```python
from build123d import *

# Parameters (mm, degrees)
SKETCH1_R           = 2.4892
BOSS_EXTRUDE1_DEPTH = 33.3375
CUT_EXTRUDE2_DEPTH  = 7.9375


with BuildPart() as part:
    # Sketch1 → Boss-Extrude1 (new, symmetric)
    with BuildSketch(Plane.XY):
        with BuildLine():
            ThreePointArc((-2.634980936, 6.35), (-3.437499983, 5.953924622), (-4.181770846, 5.456960429))
            Line((-4.181770846, 5.456960429), (-6.816751782, 0.893039571))
            ThreePointArc((-6.816751782, 0.893039571), (-6.874999966, 0), (-6.816751782, -0.893039571))
            Line((-6.816751782, -0.893039571), (-4.181770846, -5.456960429))
            ThreePointArc((-4.181770846, -5.456960429), (-3.437499983, -5.953924622), (-2.634980936, -6.35))
            Line((-2.634980936, -6.35), (2.634980936, -6.35))
            ThreePointArc((2.634980936, -6.35), (3.437499983, -5.953924622), (4.181770846, -5.456960429))
            Line((4.181770846, -5.456960429), (6.816751782, -0.893039571))
            ThreePointArc((6.816751782, -0.893039571), (6.860422465, -0.447468582), (6.874999966, 0))
            ThreePointArc((6.874999966, 0), (6.860422465, 0.447468582), (6.816751782, 0.893039571))
            Line((6.816751782, 0.893039571), (4.181770846, 5.456960429))
            ThreePointArc((4.181770846, 5.456960429), (3.437499983, 5.953924622), (2.634980936, 6.35))
            Line((2.634980936, 6.35), (-2.634980936, 6.35))
        make_face()
        Circle(SKETCH1_R, mode=Mode.SUBTRACT)
    extrude(amount=BOSS_EXTRUDE1_DEPTH, both=True)

    # Sketch2 → Cut-Extrude2 (cut)
    with BuildSketch(Plane.XY.offset(33.3375)):
        with BuildLine():
            ThreePointArc((-5.499261332, 3.174999968), (-3.175000008, 5.499261309), (1.8e-08, 6.35))
            Line((1.8e-08, 6.35), (-2.634980936, 6.35))
            ThreePointArc((-2.634980936, 6.35), (-3.437499983, 5.953924622), (-4.181770846, 5.456960429))
            Line((-4.181770846, 5.456960429), (-5.499261332, 3.174999968))
        make_face()
        with BuildLine():
            ThreePointArc((1.8e-08, 6.35), (3.175000042, 5.49926129), (5.499261354, 3.174999932))
            Line((5.499261354, 3.174999932), (4.181770846, 5.456960429))
            ThreePointArc((4.181770846, 5.456960429), (3.437499983, 5.953924622), (2.634980936, 6.35))
            Line((2.634980936, 6.35), (1.8e-08, 6.35))
        make_face()
        with BuildLine():
            ThreePointArc((5.499261354, 3.174999932), (6.133629007, 1.643500898), (6.35, 0))
            ThreePointArc((6.35, 0), (6.133629, -1.643500924), (5.499261327, -3.174999977))
            Line((5.499261327, -3.174999977), (6.816751782, -0.893039571))
            ThreePointArc((6.816751782, -0.893039571), (6.874999966, 0), (6.816751782, 0.893039571))
            Line((6.816751782, 0.893039571), (5.499261354, 3.174999932))
        make_face()
        with BuildLine():
            Line((4.181770846, -5.456960429), (5.499261327, -3.174999977))
            ThreePointArc((5.499261327, -3.174999977), (3.175000011, -5.499261308), (0, -6.35))
            Line((0, -6.35), (2.634980936, -6.35))
            ThreePointArc((2.634980936, -6.35), (3.437499983, -5.953924622), (4.181770846, -5.456960429))
        make_face()
        with BuildLine():
            Line((-2.634980936, -6.35), (0, -6.35))
            ThreePointArc((0, -6.35), (-3.174999938, -5.49926135), (-5.499261242, -3.175000124))
            Line((-5.499261242, -3.175000124), (-4.181770846, -5.456960429))
            ThreePointArc((-4.181770846, -5.456960429), (-3.437499983, -5.953924622), (-2.634980936, -6.35))
        make_face()
        with BuildLine():
            ThreePointArc((-5.499261242, -3.175000124), (-6.35, -9e-08), (-5.499261332, 3.174999968))
            Line((-5.499261332, 3.174999968), (-6.816751782, 0.893039571))
            ThreePointArc((-6.816751782, 0.893039571), (-6.874999966, 0), (-6.816751782, -0.893039571))
            Line((-6.816751782, -0.893039571), (-5.499261242, -3.175000124))
        make_face()
    cut_extrude2 = extrude(amount=-CUT_EXTRUDE2_DEPTH, mode=Mode.SUBTRACT)

    # Mirror1: Cut-Extrude2 across plane
    add(cut_extrude2.mirror(Plane.XY), mode=Mode.SUBTRACT)


solid = part.part
```
CAD build for the part. Positions are in the model's coordinates, mm. A direction names the side the tool comes from. Coordinates: 2 decimals unless noted, no trailing zeros. Write each loop counter-clockwise with the first axis right and the second up, starting at its lowest first coordinate (ties: lowest second). Pieces come first, ordered by that corner, then holes. Notation, with made-up numbers: (-24.5, -10.5) -> (1.5, -10.5) arc R34 ccw to (1.5, 25.5) -> close; hole circle Ø4 at (83.25, -1). An arc over 180 degrees is marked (long way). Return JSON: item names as keys, results as strings. Group by question number.
Q1. Drill centre lines: line 1 (X direction, y = -3.25, z = -22.5); line 2 (X direction, y = 0.75, z = 12); line 3 (Y direction, x = -2, z = -15). Where is each one in solid material? Low to high.
Q2. Cut at D-D, the plane y = 4. Give the cut face in (x, z), then the cut area to 3 significant figures.
Q3. Pull direction Y, two halves, no side cores. Call faces 1 (the face through (-3.448, -5.948, -0.356)), 2 (the face through (2.374, 0.748, -0.467)), 3 (the face through (3, 0, -33.338)): released by +Y, released by -Y, zero draft, split by the parting line, or undercut.
Q4. Cut at A-A, the plane y = 1.5. Give the cut face in (x, z), then the cut area to 3 significant figures.
Q5. Cut at B-B, the plane x = -1.5. Give the cut face in (y, z), then the cut area to 3 significant figures.
Q6. Which spindle directions (+Z, -Z, +X, -X, +Y, -Y) get a long thin tool onto all of the face, cutting with end or side? Do faces 4 (the face through (6.5, 0, 25.4)), 5 (the face through (-3, 6, 25.4)), 6 (the face through (3, -6, -25.4)), 7 (the face through (3, -6, 25.4)). Say none if no direction does.
Q7. Cut at C-C, the plane z = -1. Give the cut face in (x, y) (3 decimals), then the cut area to 3 significant figures.
Q8. Flat gauge pins, fed straight in: pin 1 (4 mm diameter, centred on x = 0, y = 0, fed in from +Z); pin 2 (3 mm diameter, centred on y = 3.5, z = 25, fed in from -X); pin 3 (6 mm diameter, centred on y = -3.5, z = 26, fed in from -X). Where does each tip first touch, or does it go through?
Returned:
{
 "1": {"line 1": "x = -5.46 to 5.46", "line 2": "x = -6.83 to -2.37, 2.37 to 6.83", "line 3": "y = -6.35 to -1.48, 1.48 to 6.35"},
 "2": {"outline": "(-5.02, -25.4) -> (-4.93, -25.4) -> (-4.93, -33.34) -> (4.93, -33.34) -> (4.93, -25.4) -> (5.02, -25.4) -> (5.02, 25.4) -> (4.93, 25.4) -> (4.93, 33.34) -> (-4.93, 33.34) -> (-4.93, 25.4) -> (-5.02, 25.4) -> close", "area": "667 mm2"},
 "3": {"face 1": "released by -Y", "face 2": "undercut", "face 3": "zero draft"},
 "4": {"outline": "(-6.47, -25.4) -> (-6.17, -25.4) -> (-6.17, -33.34) -> (-1.99, -33.34) -> (-1.99, 33.34) -> (-6.17, 33.34) -> (-6.17, 25.4) -> (-6.47, 25.4) -> close; (1.99, -33.34) -> (6.17, -33.34) -> (6.17, -25.4) -> (6.47, -25.4) -> (6.47, 25.4) -> (6.17, 25.4) -> (6.17, 33.34) -> (1.99, 33.34) -> close", "area": "588 mm2"},
 "5": {"outline": "(-6.35, -25.4) -> (-6.17, -25.4) -> (-6.17, -33.34) -> (-1.99, -33.34) -> (-1.99, 33.34) -> (-6.17, 33.34) -> (-6.17, 25.4) -> (-6.35, 25.4) -> close; (1.99, -33.34) -> (6.17, -33.34) -> (6.17, -25.4) -> (6.35, -25.4) -> (6.35, 25.4) -> (6.17, 25.4) -> (6.17, 33.34) -> (1.99, 33.34) -> close", "area": "576 mm2"},
 "6": {"face 4": "+Z, +X", "face 5": "+Z, -X, +Y", "face 6": "-Z, +X, -Y", "face 7": "+Z, +X, -Y"},
 "7": {"outline": "(-6.817, -0.893) -> (-4.182, -5.457) arc R6.875 ccw to (-2.635, -6.35) -> (2.635, -6.35) arc R6.875 ccw to (4.182, -5.457) -> (6.817, -0.893) arc R6.875 ccw to (6.817, 0.893) -> (4.182, 5.457) arc R6.875 ccw to (2.635, 6.35) -> (-2.635, 6.35) arc R6.875 ccw to (-4.182, 5.457) -> (-6.817, 0.893) arc R6.875 ccw to start; hole circle Ø4.978 at (0, 0)", "area": "118 mm2"},
 "8": {"pin 1": "passes through", "pin 2": "stops at x = -6.18", "pin 3": "stops at x = -6.85"}
}
